from build123d import *

# Parameters (mm, degrees)
SKETCH_1_R          = 14
EXTRUDE_1_DEPTH     = 14.5
SKETCH_3_R          = 7.5
EXTRUDE_3_DEPTH     = 4
SKETCH_4_R          = 1.75
CUT_EXTRUDE_1_DEPTH = 28.09704781
SKETCH_5_R          = 1
CUT_EXTRUDE_2_DEPTH = 3
SKETCH_6_R          = 1.5
CUT_EXTRUDE_3_DEPTH = 3


with BuildPart() as part:
    # 草图1 → 凸台-拉伸1 (new body)
    with BuildSketch(Plane.XY):
        with Locations(Location((0, 0, 0), (0, 0, 180))):
            Circle(SKETCH_1_R)
    extrude(amount=EXTRUDE_1_DEPTH)

    # 草图3 → 凸台-拉伸3 (add)
    with BuildSketch(Plane.XY.offset(14.5)):
        Circle(SKETCH_3_R)
    extrude(amount=EXTRUDE_3_DEPTH)

    # 草图4 → 切除-拉伸1 (cut, through all)
    with BuildSketch(Plane.XY.offset(18.5)):
        Circle(SKETCH_4_R)
    extrude(amount=-CUT_EXTRUDE_1_DEPTH, mode=Mode.SUBTRACT)

    # 草图5 → 切除-拉伸2 (cut)
    with BuildSketch(Plane.XY.offset(18.5)):
        with Locations((0, -6)):
            Circle(SKETCH_5_R)
        with Locations((-6, 0)):
            Circle(SKETCH_5_R)
        with Locations((0, 6)):
            Circle(SKETCH_5_R)
        with Locations((6, 0)):
            Circle(SKETCH_5_R)
    extrude(amount=-CUT_EXTRUDE_2_DEPTH, mode=Mode.SUBTRACT)

    # 草图6 → 切除-拉伸3 (cut)
    with BuildSketch(Plane.XY):
        with Locations((0, 8)):
            Circle(SKETCH_6_R)
        with Locations((-8, 0)):
            Circle(SKETCH_6_R)
        with Locations((0, -8)):
            Circle(SKETCH_6_R)
        with Locations((8, 0)):
            Circle(SKETCH_6_R)
    extrude(amount=CUT_EXTRUDE_3_DEPTH, mode=Mode.SUBTRACT)


solid = part.part
Model file for the job. Use its own axes, mm. A direction names the side the tool comes from. Round coordinates to 2 decimals unless told otherwise and drop trailing zeros. Loops run counter-clockwise (first coordinate to the right, second up) from the corner with the lowest first, then second, coordinate; pieces in that order, holes last. Notation, with made-up numbers: (21, 84.5) - (26, 84.5) arc R17 cw to (26, 95.5) - close; hole circle Ø5 at (4, 53). An arc over 180 degrees is marked (long way). Write each question's results on one line, items separated by ' | '.
(1) Mould opens along X. For faces 4 (the cylindrical face through (-0.325, 6.536, 1.479)), 5 (the cylindrical face through (-12.932, 5.362, 7.148)), 6 (the flat face through (-6, 6, 14.5)) say: released by +X, released by -X, zero draft, split by the parting line, or undercut.
Answer below:
face 4: undercut | face 5: split by the parting line | face 6: zero draft
(2) Saw through at D-D, the plane z = 7.25. List the corners of the cut face in (x, y), then the cut area to 3 significant figures.
Answer below:
outline: circle Ø28 at (0, 0); hole circle Ø3.5 at (0, 0) | area: 606 mm^2
(3) Saw through at C-C, the plane x = -8. List the corners of the cut face in (y, z), then the cut area to 3 significant figures.
Answer below:
outline: (-11.49, 0) - (-1.5, 0) - (-1.5, 3) - (1.5, 3) - (1.5, 0) - (11.49, 0) - (11.49, 14.5) - (-11.49, 14.5) - close | area: 324 mm^2
(4) Saw through at B-B, the plane z = 1.75. List the corners of the cut face in (x, y).
Answer below:
outline: circle Ø28 at (0, 0); hole circle Ø3 at (-8, 0); hole circle Ø3.5 at (0, 0); hole circle Ø3 at (0, -8); hole circle Ø3 at (0, 8); hole circle Ø3 at (8, 0)
(5) Wall check: L1, parallel to Y at x = 0, z = 16.45; L2, parallel to Y at x = 0, z = 12; L3, parallel to Y at x = -0.5, z = 16.5. Give the ranges that are in metal, low to high.
Answer below:
L1: y = -7.5 to -7, -5 to -1.75, 1.75 to 5, 7 to 7.5 | L2: y = -14 to -1.75, 1.75 to 14 | L3: y = -7.48 to -6.87, -5.13 to -1.68, 1.68 to 5.13, 6.87 to 7.48
(6) 3-axis set-ups, long thin cutter, end or side, ignore diameter. For faces 1 (the cylindrical face through (-6.8, -0.6, 17)), 2 (the flat face through (2, -2, 18.5)), 3 (the flat face through (8, 0, 3)): which of +Z, -Z, +X, -X, +Y, -Y reach the whole face in a straight line?
Answer below:
face 1: +Z | face 2: +Z, +X, -X, +Y, -Y | face 3: -Z
(7) Saw through at A-A, the plane y = 0. List the corners of the cut face in (x, z), then the cut area to 3 significant figures.
Answer below:
outline: (-14, 0) - (-9.5, 0) - (-9.5, 3) - (-6.5, 3) - (-6.5, 0) - (-1.75, 0) - (-1.75, 18.5) - (-5, 18.5) - (-5, 15.5) - (-7, 15.5) - (-7, 18.5) - (-7.5, 18.5) - (-7.5, 14.5) - (-14, 14.5) - close; (1.75, 0) - (6.5, 0) - (6.5, 3) - (9.5, 3) - (9.5, 0) - (14, 0) - (14, 14.5) - (7.5, 14.5) - (7.5, 18.5) - (7, 18.5) - (7, 15.5) - (5, 15.5) - (5, 18.5) - (1.75, 18.5) - close | area: 371 mm^2
(8) Pin check, flat tips, straight feed: pin 1 (3 mm diameter, centred on x = -10, y = 7, fed in from +Z); pin 2 (1.5 mm diameter, centred on y = -9, z = 10.5, fed in from +X); pin 3 (1.6 mm diameter, centred on x = 0, y = 6, fed in from +Z). Stop position of each tip, or through.
Answer below:
pin 1: stops at z = 14.5 | pin 2: stops at x = 11.31 | pin 3: stops at z = 15.5
